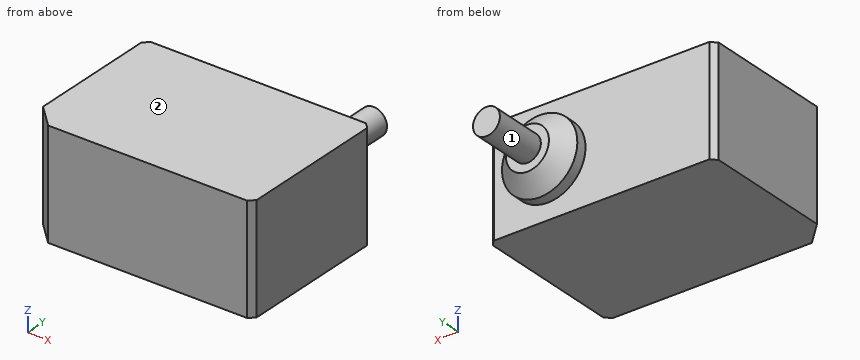
from build123d import *

# Parameters (mm, degrees)
SKETCH1_W           = 42
SKETCH1_H           = 29
BOSS_EXTRUDE1_DEPTH = 20
CHAMFER1_SIZE       = 4
CHAMFER2_SIZE       = 1
CHAMFER3_SIZE       = 1
SKETCH4_R           = 7
BOSS_EXTRUDE2_DEPTH = 5
CHAMFER4_SIZE       = 3
SKETCH5_R           = 2.5
BOSS_EXTRUDE3_DEPTH = 10


with BuildPart() as part:
    # Sketch1 → Boss-Extrude1 (new body)
    with BuildSketch(Plane.XY):
        with Locations((21, 14.5)):
            Rectangle(SKETCH1_W, SKETCH1_H)
    extrude(amount=BOSS_EXTRUDE1_DEPTH)

    # Chamfer1
    chamfer1_edges = [part.edges().sort_by_distance(p)[0] for p in [
        (0, 0, 10),
    ]]
    chamfer(chamfer1_edges, length=CHAMFER1_SIZE)

    # Chamfer2
    chamfer2_edges = [part.edges().sort_by_distance(p)[0] for p in [
        (0, 29, 10),
        (42, 29, 10),
    ]]
    chamfer(chamfer2_edges, length=CHAMFER2_SIZE)

    # Chamfer3
    chamfer3_edges = [part.edges().sort_by_distance(p)[0] for p in [
        (42, 0, 10),
    ]]
    chamfer(chamfer3_edges, length=CHAMFER3_SIZE)

    # Sketch4 → Boss-Extrude2 (add)
    with BuildSketch(Plane(origin=(0, 29, 0), x_dir=(1, 0, 0), z_dir=(0, 1, 0))):
        with Locations(Location((31, -10, 0), (0, 0, 90))):
            Circle(SKETCH4_R)
    extrude(amount=BOSS_EXTRUDE2_DEPTH)

    # Chamfer4
    chamfer4_edges = [part.edges().sort_by_distance(p)[0] for p in [
        (31, 34, 17),
    ]]
    chamfer(chamfer4_edges, length=CHAMFER4_SIZE)

    # Sketch5 → Boss-Extrude3 (add)
    with BuildSketch(Plane(origin=(0, 34, 0), x_dir=(1, 0, 0), z_dir=(0, 1, 0))):
        with Locations(Location((31, -10, 0), (0, 0, 270))):
            Circle(SKETCH5_R)
    extrude(amount=BOSS_EXTRUDE3_DEPTH)


solid = part.part
CAD build for the part. Positions are in the model's coordinates, mm. Face numbers are marked on the shaded views. A direction names the side the tool comes from. Give positions to 0.01 mm unless a question says otherwise; leave off trailing zeros. Order: outer loops, then holes, each group sorted by start corner. A loop starts at its lowest first (then second) coordinate and runs counter-clockwise, first axis right, second up. Notation, with made-up numbers: (-29.75, 9) - (10.25, 9) arc R20 ccw to (10.25, 22) - close; hole circle Ø5 at (66.5, 25.25). An arc over 180 degrees is marked (long way). Answer in a Markdown table with one row per item.
1. Saw through at A-A, the plane x = 31. Give the cut face in (y, z), plus the area to 3 significant figures.
Data:
| item | result |
|---|---|
| outline | (0, 0) - (29, 0) - (29, 3) - (31, 3) - (34, 6) - (34, 7.5) - (44, 7.5) - (44, 12.5) - (34, 12.5) - (34, 14) - (31, 17) - (29, 17) - (29, 20) - (0, 20) - close |
| area | 691 mm² |
2. Saw through at B-B, the plane z = 10. Give the cut face in (x, y).
Data:
| item | result |
|---|---|
| outline | (0, 4) - (4, 0) - (41, 0) - (42, 1) - (42, 28) - (41, 29) - (38, 29) - (38, 31) - (35, 34) - (33.5, 34) - (33.5, 44) - (28.5, 44) - (28.5, 34) - (27, 34) - (24, 31) - (24, 29) - (1, 29) - (0, 28) - close |
3. Saw through at C-C, the plane y = 39. Give the cut face in (x, z).
Data:
| item | result |
|---|---|
| outline | circle Ø5 at (31, 10) |
4. Tool access for the marked faces 1 and 2: list every direction of +Z, -Z, +X, -X, +Y, -Y with a clear straight run to the whole face (end or side of a thin tool).
Data:
| item | result |
|---|---|
| face 1 | +Y |
| face 2 | +Z, +X, -X, +Y, -Y |
5. Saw through at D-D, the plane x = 6.5. Give the cut face in (y, z).
Data:
| item | result |
|---|---|
| outline | (0, 0) - (29, 0) - (29, 20) - (0, 20) - close |
6. Probe probe 1 along Y at (x, z) = (34, 10.5); probe 2 along Y at (x, z) = (26, 18); probe 3 along X at (y, z) = (31.5, 9.5). List the from-to ranges inside material, lowest first. Write a range as [from, to].
Data:
| item | result |
|---|---|
| probe 1 | y = [0, 34] |
| probe 2 | y = [0, 29] |
| probe 3 | x = [24.52, 37.48] |
7. Flat gauge pins, fed straight in: pin 1 (2 mm diameter, centred on x = 22, y = 31, fed in from +Z) (3 decimals); pin 2 (3 mm diameter, centred on x = 15, z = 13.5, fed in from +Y); pin 3 (10 mm diameter, centred on x = 23, z = 14.5, fed in from +Y). Where does each tip first touch, or does it go through?
Data:
| item | result |
|---|---|
| pin 1 | passes through |
| pin 2 | stops at y = 29 |
| pin 3 | stops at y = 33.82 |
